Could you check a few things on this model? Use its own coordinates, in mm. A direction names the side the tool comes from. Give positions to 0.01 mm unless a question says otherwise; leave off trailing zeros. Loops run counter-clockwise (first coordinate to the right, second up) from the corner with the lowest first, then second, coordinate; pieces in that order, holes last. Notation, with made-up numbers: M 36.5,-9.5 L 68.5,-9.5 A19 ccw 68.5,7.5 Z; hole C 28,55 d10. An arc over 180 degrees is marked long. Answer in a Markdown table with one row per item. Add a question column.
1. If we section it at D-D on x = 3.25: List the corners of the cut face in (y, z) for me.
2. If we section it at C-C on y = 20: List the corners of the cut face in (x, z) for me (1 decimal).
3. Thinking about a two-plate mould opening in Y: for faces 1 (the flat face through (0, 12, -1.887)), 2 (the flat face through (3, 19.5, 3)), 3 (the flat face through (4, 0, 3)), 4 (the flat face through (2, 22, 5.553)), which applies, released by +Y, released by -Y, zero draft, split by the parting line, or undercut?
4. Which directions (+Z, -Z, +X, -X, +Y, -Y) give clear straight access to the entire face, cutting with the end or side of a thin tool? Please do faces 5 (the flat face through (4, 4.5, 3)), 6 (the flat face through (-3.254, 22, 4)), 7 (the flat face through (4, 24, 3)).
5. I'm going to push flat-ended pins straight in: pin 1 Ø1.5 at (x, z) = (-2, 1.5) entering from -Y; pin 2 Ø0.8 at (y, z) = (2, 4.5) entering from -X; pin 3 Ø4.5 at (x, y) = (0.5, 9.5) entering from +Z. Where does each tip first touch, or does it pass through?
6. If we section it at B-B on z = -0.5: List the corners of the cut face in (x, y) for me (3 decimals), then the cut area to 3 significant figures.
7. I need wall thicknesses on line 1 along Y through (x, z) = (-3, 4); line 2 along Z through (x, y) = (0, 15.5); line 3 along X through (y, z) = (21.75, 4) (3 decimals). Which ranges of each line are inside material? Lowest first, please. Write a range as from..to.
8. If we section it at A-A on x = 5.25: List the corners of the cut face in (y, z) for me.
Solid Edge part; units mm, degrees
sketch "Sketch1" plane through (0, 0, 0) normal (0, -1, 0) x (1, 0, 0)
  line L0 (7.725, 5.5532) -> (-3.2544, 5.5532)
  line L1 (-3.2544, 5.5532) -> (-3.2544, 2.8412)
  line L2 (-3.2544, 2.8412) -> (2.1676, 2.65)
  arc A0 (2.1676, 2.65) -> (2.2221, -1.8869) centre (2.2221, 0.3819) cw
  line L3 (-7.8594, -1.8869) -> (2.2221, -1.8869)
  line L4 (-7.8594, -1.8869) -> (-7.8594, -3.2075)
  line L5 (-7.8594, -3.2075) -> (7.725, -3.2075)
  line L6 (7.725, -3.2075) -> (7.725, 5.5532)
extrude "Protrusion1" add sketch "Sketch1" against normal blind 24
sketch "Sketch2" plane through (4.513, 12, 5.5532) normal (0, 0, 1) x (1, 0, 0)
  line L0 (-20.7401, 7.5) -> (6.9953, 7.5)
  line L1 (6.9953, 7.5) -> (6.9953, -7.5)
  line L2 (6.9953, -7.5) -> (-20.7401, -7.5)
  line L3 (-20.7401, -7.5) -> (-20.7401, 7.5)
extrude "Cutout1" cut sketch "Sketch2" against normal up to vertex (7.4402 mm away)
Results:
| question | item | result |
|---|---|---|
| 1 | outline | M 0,-3.21 L 24,-3.21 L 24,-1.64 L 19.5,-1.64 L 19.5,-1.89 L 4.5,-1.89 L 4.5,-1.64 L 0,-1.64 Z; M 0,2.4 L 4.5,2.4 L 4.5,5.55 L 0,5.55 Z; M 19.5,2.4 L 24,2.4 L 24,5.55 L 19.5,5.55 Z |
| 2 | outline | M -7.9,-3.2 L 7.7,-3.2 L 7.7,5.6 L -3.3,5.6 L -3.3,2.8 L 2.2,2.7 A2.3 cw long 2.2,-1.9 L -7.9,-1.9 Z |
| 3 | face 1 | undercut |
| 3 | face 2 | undercut |
| 3 | face 3 | released by -Y |
| 3 | face 4 | zero draft |
| 4 | face 5 | +Z, +X, -X |
| 4 | face 6 | +Z, -X, +Y, -Y |
| 4 | face 7 | +Z, -Z, +X, -X, +Y |
| 5 | pin 1 | through |
| 5 | pin 2 | x = -3.25 |
| 5 | pin 3 | z = -1.89 |
| 6 | outline | M 4.312,0 L 7.725,0 L 7.725,4.5 L 4.312,4.5 Z; M 4.312,19.5 L 7.725,19.5 L 7.725,24 L 4.312,24 Z |
| 6 | area | 30.7 mm2 |
| 7 | line 1 | 0..4.5, 19.5..24 |
| 7 | line 2 | -3.21..-1.89 |
| 7 | line 3 | -3.254..7.725 |
| 8 | outline | M 0,-3.21 L 24,-3.21 L 24,5.55 L 19.5,5.55 L 19.5,-1.89 L 4.5,-1.89 L 4.5,5.55 L 0,5.55 Z |
